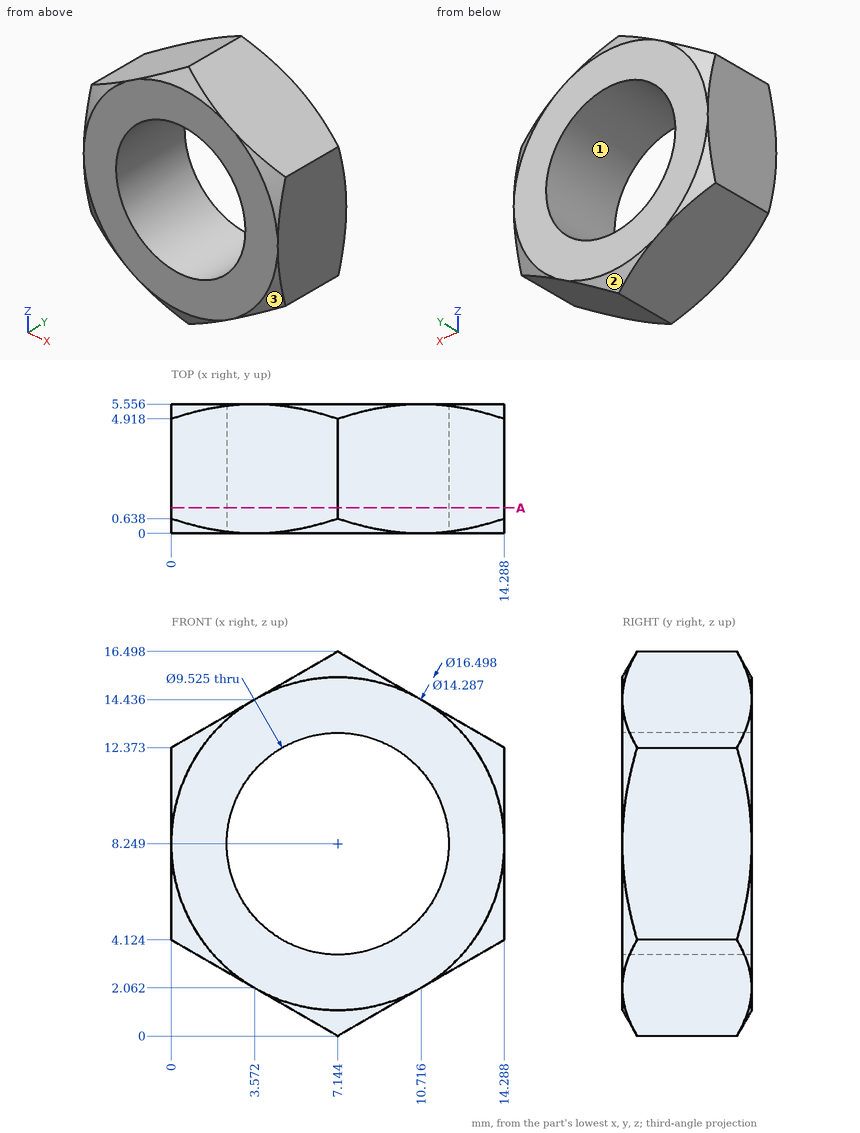
Can you work these out from the drawing? Everything is in mm from the part's minimum corner. Give positions to 0.01 mm unless a question says otherwise; leave off trailing zeros. Order: outer loops, then holes, each group sorted by start corner. A loop starts at its lowest first (then second) coordinate and runs counter-clockwise, first axis right, second up. Notation, with made-up numbers: M -22.5,0 L 18.5,0 A13 ccw 18.5,12 Z; hole C -37.5,33.25 d8. An arc over 180 degrees is marked long. Use a Markdown table: item, result. Add a question column.
1. If we mould it in two halves opening along X, with no side actions, what happens to the marked faces 1, 2 and 3? For each: +X half, -X half, draft (parallel to the pull), parting line (faces both ways), or undercut.
2. Suppose I cut it at A-A (y = 1.1). List the corners of the cut face in (x, z) for me (1 decimal).
3. I need wall thicknesses on probe 1 along Z at (x, y) = (10.5, 1.25) (1 decimal); probe 2 along X at (y, z) = (3.65, 12.5) (1 decimal); probe 3 along X at (y, z) = (1.1, 9.75) (1 decimal). Which ranges of each line are inside material? Lowest first, please. Write a range as from..to.
Results list:
| question | item | result |
|---|---|---|
| 1 | face 1 | undercut |
| 1 | face 2 | parting line |
| 1 | face 3 | +X half |
| 2 | outline | M 0,4.1 L 7.1,0 L 14.3,4.1 L 14.3,12.4 L 7.1,16.5 L 0,12.4 Z; hole C 7.1,8.2 d9.5 |
| 3 | probe 1 | z = 1.9..4.9, 11.6..14.6 |
| 3 | probe 2 | x = 0.2..5, 9.3..14.1 |
| 3 | probe 3 | x = 0..2.6, 11.7..14.3 |
